Build history of the part. All positions in model axes, mm. A direction names the side the tool comes from. Round coordinates to 2 decimals unless told otherwise and drop trailing zeros. Write each loop counter-clockwise with the first axis right and the second up, starting at its lowest first coordinate (ties: lowest second). Pieces come first, ordered by that corner, then holes.
Autodesk Fusion 360 part; units mm, degrees
sketch "Sketch1" plane through (0, 0, 0) normal (0, 0, 1) x (1, 0, 0)
  line L0 (-160.2344, 10.4731) -> (19.7656, 10.4731)
  line L1 (19.7656, 10.4731) -> (19.7656, -169.5269)
  line L2 (19.7656, -169.5269) -> (-160.2344, -169.5269)
  line L3 (-160.2344, -169.5269) -> (-160.2344, 10.4731)
  dimension "d1" = 180
  dimension "d2" = 180
extrude "Extrude1" add sketch "Sketch1" along normal blind 10
sketch "Sketch2" plane through (0, 0, 10) normal (0, 0, 1) x (-1, 0, 0)
  line L0 (160.2344, 169.5269) -> (-19.7656, 169.5269)
  line L1 (-19.7656, 169.5269) -> (-19.7656, -10.4731)
  line L2 (-19.7656, -10.4731) -> (160.2344, -10.4731)
  line L3 (160.2344, -10.4731) -> (160.2344, 169.5269)
  line L4 (160.2344, 59.5269) -> (140.2344, 59.5269)
  line L5 (140.2344, 59.5269) -> (140.2344, 99.5269)
  line L6 (140.2344, 99.5269) -> (160.2344, 99.5269)
  line L7 (160.2344, 99.5269) -> (160.2344, 59.5269)
  line L8 (0.2344, 59.5269) -> (-19.7656, 59.5269)
  line L9 (-19.7656, 59.5269) -> (-19.7656, 99.5269)
  line L10 (-19.7656, 99.5269) -> (0.2344, 99.5269)
  line L11 (0.2344, 99.5269) -> (0.2344, 59.5269)
  line L12 (90.2344, -10.4731) -> (50.2344, -10.4731)
  line L13 (50.2344, -10.4731) -> (50.2344, 9.5269)
  line L14 (50.2344, 9.5269) -> (90.2344, 9.5269)
  line L15 (90.2344, 9.5269) -> (90.2344, -10.4731)
  line L16 (90.2344, 149.5269) -> (50.2344, 149.5269)
  line L17 (50.2344, 149.5269) -> (50.2344, 169.5269)
  line L18 (50.2344, 169.5269) -> (90.2344, 169.5269)
  line L19 (90.2344, 169.5269) -> (90.2344, 149.5269)
  dimension "d5" = 20
  dimension "d6" = 20
  dimension "d7" = 20
  dimension "d8" = 20
  dimension "d9" = 40
  dimension "d10" = 40
  dimension "d11" = 40
  dimension "d12" = 40
  dimension "d13" = 70
  dimension "d14" = 70
  dimension "d15" = 70
  dimension "d16" = 70
extrude "Extrude2" add sketch "Sketch2" along normal blind 30 contours L0 L16 L17 L18 L19 | L3 L4 L5 L6 L7 | L1 L8 L9 L10 L11 | L2 L12 L13 L14 L15
sketch "Sketch3" plane through (19.7656, 0, 0) normal (1, 0, 0) x (0, 1, 0)
  line L0 (-169.5269, 0) -> (10.4731, 0)
  line L1 (10.4731, 0) -> (10.4731, 10)
  line L2 (10.4731, 10) -> (-59.5269, 10)
  line L3 (-59.5269, 10) -> (-59.5269, 40)
  line L4 (-59.5269, 40) -> (-99.5269, 40)
  line L5 (-99.5269, 40) -> (-99.5269, 10)
  line L6 (-99.5269, 10) -> (-169.5269, 10)
  line L7 (-169.5269, 10) -> (-169.5269, 0)
  circle A0 centre (-79.5269, 22) radius 6 construction
  line L8 (-74.5269, 29.5) -> (-84.5269, 29.5) construction
  line L9 (-84.5269, 29.5) -> (-84.5269, 15.25) construction
  line L10 (-83.7769, 14.5) -> (-75.2769, 14.5) construction
  line L11 (-74.5269, 15.25) -> (-74.5269, 29.5) construction
  line L12 (-74.5269, 29.5) -> (-84.5269, 14.5) construction
  line L13 (-84.5269, 29.5) -> (-74.5269, 14.5) construction
  line L14 (-83.7769, 14.5) -> (-84.5269, 15.25)
  line L15 (-75.2769, 14.5) -> (-74.5269, 15.25)
  line L16 (-83.839, 14.35) -> (-75.2147, 14.35)
  line L17 (-75.2147, 14.35) -> (-74.3769, 15.1879)
  line L18 (-74.3769, 15.1879) -> (-74.3769, 29.65)
  line L19 (-74.3769, 29.65) -> (-84.6769, 29.65)
  line L20 (-84.6769, 29.65) -> (-84.6769, 15.1879)
  line L21 (-83.839, 14.35) -> (-84.6769, 15.1879)
  point P0 (-79.5269, 22)
  dimension "d19" = 12
  dimension "d20" = 18
  dimension "d21" = 20
  dimension "d36" = 10
  dimension "d37" = 15
  dimension "d38" = 0.15
  dimension "d39" = 0.75
  dimension "d40" = 0.75
  dimension "d41" = 0.75
  dimension "d42" = 0.75
extrude "Extrude3" cut sketch "Sketch3" against normal blind 30 contours L16 L17 L18 L19 L20 L21
ref_plane "WorkPlane1" through (-70.2344, -79.5269, 20) normal (0, -1, 0) x (1, 0, 0)
ref_plane "WorkPlane2" through (-70.2344, -79.5269, 20) normal (1, 0, 0) x (0, 1, 0)
pattern_circular "C-Pattern1" count 4 over 360 about axis through (-70.2344, -79.5269, -13.6) along (0, 0, 1) of "Extrude3"
sketch "Sketch4" plane through (0, -59.5269, 0) normal (0, 1, 0) x (-1, 0, 0)
  line L0 (-19.7656, 10) -> (0.2344, 10)
  line L1 (0.2344, 10) -> (0.2344, 40)
  line L2 (0.2344, 40) -> (-19.7656, 40)
  line L3 (-19.7656, 40) -> (-19.7656, 10)
  circle A0 centre (-9.7656, 22) radius 3.1
  dimension "d26" = 6.2
  dimension "d27" = 18
  dimension "d28" = 10
extrude "Extrude4" cut sketch "Sketch4" against normal blind 20 contours A0
pattern_circular "C-Pattern2" count 4 over 360 about axis through (-70.2344, -79.5269, -13.6) along (0, 0, 1) of "Extrude4"
chamfer "Chamfer1" distance 1 angle 45 16 edges at (-0.2344, -79.5269, 40) (9.7656, -99.5269, 40) (19.7656, -79.5269, 40) (9.7656, -59.5269, 40) (-70.2344, 10.4731, 40) (-70.2344, -9.5269, 40) (-50.2344, 0.4731, 40) (-90.2344, 0.4731, 40) (-150.2344, -59.5269, 40) (-140.2344, -79.5269, 40) (-160.2344, -79.5269, 40) (-150.2344, -99.5269, 40) (-90.2344, -159.5269, 40) (-70.2344, -149.5269, 40) (-70.2344, -169.5269, 40) (-50.2344, -159.5269, 40)
chamfer "Chamfer2" distance 2 angle 45 12 edges at (-140.2344, -79.5269, 10) (-150.2344, -99.5269, 10) (-150.2344, -59.5269, 10) (-70.2344, -149.5269, 10) (-90.2344, -159.5269, 10) (-90.2344, 0.4731, 10) (-70.2344, -9.5269, 10) (-0.2344, -79.5269, 10) (9.7656, -99.5269, 10) (-50.2344, -159.5269, 10) (9.7656, -59.5269, 10) (-50.2344, 0.4731, 10)
chamfer "Chamfer3" distance 2 angle 45 8 edges at (-126.2344, 10.4731, 10) (-160.2344, -23.5269, 10) (19.7656, -23.5269, 10) (19.7656, -135.5269, 10) (-14.2344, -169.5269, 10) (-14.2344, 10.4731, 10) (-126.2344, -169.5269, 10) (-160.2344, -135.5269, 10)
equation "d40 = d39"
equation "d42 = d41"
1) Mould opens along Y. For faces 6 (the flat face through (10, -80, 14.35)), 7 (the flat face through (-0.234, -80, 31)), 8 (the flat face through (8.92, -100.61, 10.917)) say: released by +Y, released by -Y, zero draft, split by the parting line, or undercut.
Results:
face 6: undercut
face 7: zero draft
face 8: released by -Y
2) Slice it at D-D (x = -29.5). Write the cut outline in (y, z), plus the area to 3 significant figures.
Results:
outline: (-169.53, 0) - (10.47, 0) - (10.47, 8) - (8.47, 10) - (-167.53, 10) - (-169.53, 8) - close
area: 1,800 mm2
3) Slice it at C-C (y = -17). Write the cut outline in (x, z).
Results:
outline: (-160.23, 0) - (19.77, 0) - (19.77, 8) - (17.77, 10) - (-158.23, 10) - (-160.23, 8) - close
4) Slice it at A-A (y = -87). Write the cut outline in (x, z), plus the area to 3 significant figures.
Results:
outline: (-160.23, 0) - (19.77, 0) - (19.77, 39) - (18.77, 40) - (0.77, 40) - (-0.23, 39) - (-0.23, 12) - (-2.23, 10) - (-138.23, 10) - (-140.23, 12) - (-140.23, 39) - (-141.23, 40) - (-159.23, 40) - (-160.23, 39) - close; hole circle Ø6.2 at (-150.23, 22)
area: 2,970 mm2
5) Slice it at B-B (x = -59). Write the cut outline in (y, z).
Results:
outline: (-169.53, 0) - (10.47, 0) - (10.47, 39) - (9.47, 40) - (-8.53, 40) - (-9.53, 39) - (-9.53, 12) - (-11.53, 10) - (-147.53, 10) - (-149.53, 12) - (-149.53, 39) - (-150.53, 40) - (-168.53, 40) - (-169.53, 39) - close; hole circle Ø6.2 at (-159.53, 22)
6) Pin check, flat tips, straight feed: pin 1 Ø1 at (y, z) = (-151, 14) entering from -X; pin 2 Ø11.5 at (x, z) = (-153, 19.5) entering from -Y; pin 3 Ø22 at (x, z) = (-153.5, 27) entering from +Y; pin 4 Ø8 at (y, z) = (-74.5, 23) entering from -X. Stop position of each tip, or through.
Results:
pin 1: stops at x = -90.23
pin 2: stops at y = -99.53
pin 3: stops at y = -59.53
pin 4: stops at x = -160.23
7) Wall check: L1, parallel to X at y = -64.5, z = 28; L2, parallel to Y at x = -143.5, z = 27; L3, parallel to Z at x = -53, y = -128.5. Give the ranges that are in metal, low to high.
Results:
L1: x = -160.23 to -140.23, -0.23 to 19.77
L2: y = -99.53 to -84.68, -74.38 to -59.53
L3: z = 0 to 10
8) Which spindle directions (+Z, -Z, +X, -X, +Y, -Y) get a long thin tool onto all of the face, cutting with end or side? Do faces 1 (the flat face through (-71, -149.527, 31)), 2 (the flat face through (-71, -78, 10)), 3 (the flat face through (-50.234, -159.4, 25.3)), 4 (the flat face through (10, -79, 29.65)), 5 (the flat face through (-75.384, -160, 23)). Say none if no direction does.
Results:
face 1: +Z, +X, -X
face 2: +Z
face 3: +Z, +X, +Y, -Y
face 4: +X, -X
face 5: +Y, -Y
